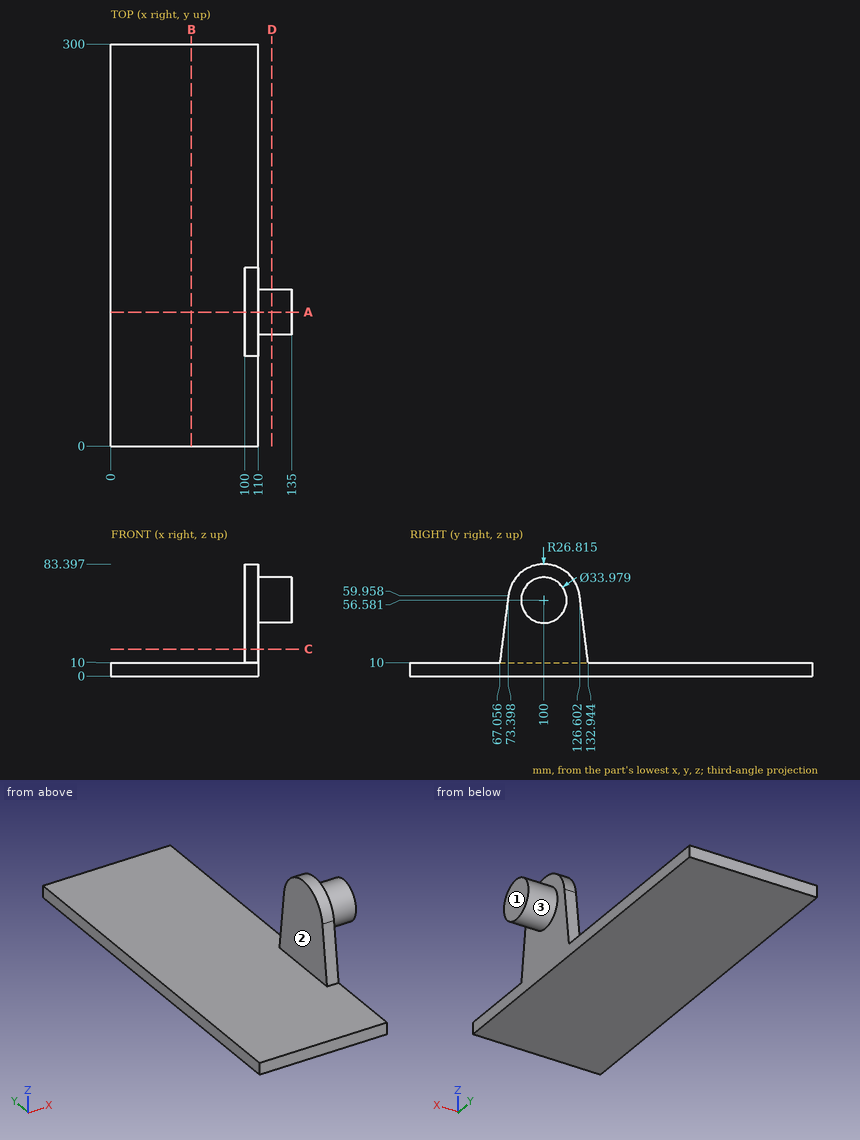
Check sheet for the drawn part. Datum: minimum x, y, z corner. Units: mm. A direction names the side the tool comes from. Coordinates: 2 decimals unless noted, no trailing zeros. Loops run counter-clockwise (first coordinate to the right, second up) from the corner with the lowest first, then second, coordinate; pieces in that order, holes last. Notation, with made-up numbers: (32, 72.25) -> (61, 72.25) arc R32 ccw to (61, 105.25) -> close; hole circle Ø11 at (16.5, 49). An arc over 180 degrees is marked (long way). Answer as CSV lines item,"result".
1) Cross-section at A-A, the plane y = 100. Record the cut outline in (x, z).
Found:
outline,"(0, 0) -> (110, 0) -> (110, 39.59) -> (135, 39.59) -> (135, 73.57) -> (110, 73.57) -> (110, 83.4) -> (100, 83.4) -> (100, 10) -> (0, 10) -> close"
2) Tool access check on the marked faces 1, 2 and 3. Record the directions out of +Z, -Z, +X, -X, +Y, -Y that give a thin tool (end or side, any length) a straight path to the whole face; none if there is none.
Found:
face 1,"+Z, -Z, +X, +Y, -Y"
face 2,"+Z, -X, +Y, -Y"
face 3,"+X"
3) Depth check by flat-ended pin: pin 1 (10 mm diameter, centred on y = 91, z = 29.5, fed in from -X); pin 2 (6 mm diameter, centred on x = 24.5, y = 35.5, fed in from +Z). Enter the tip coordinate at first touch or a pass-through.
Found:
pin 1,"stops at x = 100"
pin 2,"stops at z = 10"
4) Cross-section at D-D, the plane x = 120. Record the cut outline in (y, z).
Found:
outline,"circle Ø33.98 at (100, 56.58)"
5) Cross-section at C-C, the plane z = 20. Record the cut outline in (x, y) (1 decimal).
Found:
outline,"(100, 68.3) -> (110, 68.3) -> (110, 131.7) -> (100, 131.7) -> close"
6) Thickness scan on L1, parallel to X at y = 114, z = 75.5; L2, parallel to Z at x = 69.5, y = 268; L3, parallel to Y at x = 106, z = 19. Record the ranges inside material, lowest first. Write a range as from..to.
Found:
L1,"x = 100..110"
L2,"z = 0..10"
L3,"y = 68.2..131.8"
7) Cross-section at B-B, the plane x = 60. Record the cut outline in (y, z), then the cut area to 3 significant figures.
Found:
outline,"(0, 0) -> (300, 0) -> (300, 10) -> (0, 10) -> close"
area,"3,000 mm2"
